```python
from build123d import *

# Parameters (mm, degrees)
SCHIZZO1_R                   = 2.5
ESTRUSIONE_ESTRUSIONE1_DEPTH = 100
SCHIZZO2_R                   = 0.5
TAGLIO_ESTRUSIONE1_DEPTH     = 3.5
SCHIZZO3_R                   = 0.5
TAGLIO_ESTRUSIONE2_DEPTH     = 3.5000001


with BuildPart() as part:
    # Schizzo1 → Estrusione-Estrusione1 (new body)
    with BuildSketch(Plane.XY):
        Circle(SCHIZZO1_R)
    extrude(amount=ESTRUSIONE_ESTRUSIONE1_DEPTH)

    # Schizzo2 → Taglio-Estrusione1 (cut, through all)
    with BuildSketch(Plane(origin=(0, 0, 0), x_dir=(1, 0, 0), z_dir=(0, 1, 0))):
        with Locations((0, -1)):
            Circle(SCHIZZO2_R)
    extrude(amount=-TAGLIO_ESTRUSIONE1_DEPTH, mode=Mode.SUBTRACT)

    # Schizzo3 → Taglio-Estrusione2 (cut, through all)
    with BuildSketch(Plane(origin=(0, 0, 0), x_dir=(1, 0, 0), z_dir=(0, 1, 0))):
        with Locations((0, -99)):
            Circle(SCHIZZO3_R)
    extrude(amount=-TAGLIO_ESTRUSIONE2_DEPTH, mode=Mode.SUBTRACT)


solid = part.part
```
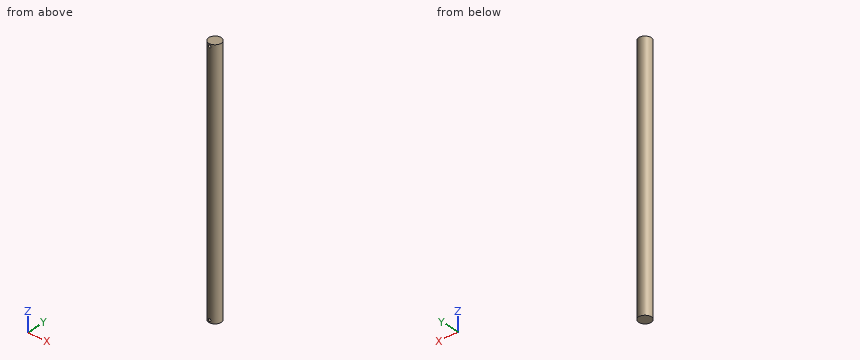
The model under review builds one solid part; all positions refer to its coordinate system, in mm. Round coordinates to 2 decimals unless told otherwise and drop trailing zeros. Loops run counter-clockwise (first coordinate to the right, second up) from the corner with the lowest first, then second, coordinate; pieces in that order, holes last.
Item 1: Take a section at A-A (y = -1.6). Write out the cut boundary in (x, z), then the cut area to 3 significant figures.
Determined:
outline: (-1.92, 0) - (1.92, 0) - (1.92, 100) - (-1.92, 100) - close; hole circle Ø1 at (0, 1); hole circle Ø1 at (0, 99)
area: 383 mm2
Item 2: Take a section at C-C (x = -1.4). Write out the cut boundary in (y, z).
Determined:
outline: (-2.07, 0) - (2.07, 0) - (2.07, 100) - (-2.07, 100) - close
Item 3: For line 1 (Z direction, x = 0, y = -1.35); line 2 (Y direction, x = -0.1, z = 21); line 3 (Z direction, x = 0.3, y = -1.3), list the stretches that pass through material, from the lowest coordinate up.
Determined:
line 1: z = 0 to 0.5, 1.5 to 98.5, 99.5 to 100
line 2: y = -2.5 to 2.5
line 3: z = 0 to 0.6, 1.4 to 98.6, 99.4 to 100
Item 4: Take a section at B-B (z = 35). Write out the cut boundary in (x, y).
Determined:
outline: circle Ø5 at (0, 0)
Item 5: Clearance check with flat-ended pins moving along their axes: pin 1 Ø0.5 at (x, z) = (0, 99) entering from -Y; pin 2 Ø1 at (x, z) = (1.5, 79.5) entering from -Y. State where each tip first meets the part, or that it passes through.
Determined:
pin 1: stops at y = 0
pin 2: stops at y = -2.29
